Source: CAD feature listing. Evaluate the final solid. Frame: model axes, mm. Round coordinates to 2 decimals unless told otherwise and drop trailing zeros. Loops run counter-clockwise (first coordinate to the right, second up) from the corner with the lowest first, then second, coordinate; pieces in that order, holes last.
(1) Material intervals for probe 1 along Z at (x, y) = (0.2, -16.5) (3 decimals); probe 2 along Z at (x, y) = (0.85, -91.5) (3 decimals); probe 3 along Y at (x, z) = (1.05, -136), sorted ascending.
(2) Section C-C, the plane y = -9. Return the cut outline in (x, z) (3 decimals), plus the area to 3 significant figures.
(3) First-contact query: pin 1 Ø0.8 at (x, z) = (0.5, -54) entering from -Y (3 decimals); pin 2 Ø0.8 at (x, y) = (1, 13) entering from +Z (3 decimals); pin 3 Ø0.5 at (x, z) = (1, -14) entering from +Y (3 decimals). Flat tips, straight axial feed; report the tip coordinate or a pass-through.
(4) Section B-B, the plane z = -36. Return the cut outline in (x, y), plus the area to 3 significant figures.
(5) Section A-A, the plane x = 0.3. Return the cut outline in (y, z) (1 decimal).
Autodesk Inventor part; units mm, degrees
ref_plane "YZ Plane" through (0, 0, 0) normal (1, 0, 0) x (0, 1, 0)
ref_plane "XZ Plane" through (0, 0, 0) normal (0, 1, 0) x (-1, 0, 0)
ref_plane "XY Plane" through (0, 0, 0) normal (0, 0, 1) x (1, 0, 0)
sketch "Key" plane through (0, 0, 0) normal (0, 0, 1) x (1, 0, 0)
  line L0 (-9.525, 9.525) -> (9.525, 9.525) construction
  line L1 (9.525, 9.525) -> (9.525, -9.525) construction
  line L2 (9.525, -9.525) -> (-9.525, -9.525) construction
  line L3 (-9.525, -9.525) -> (-9.525, 9.525) construction
  line L4 (-9.525, 9.525) -> (9.525, -9.525) construction
  line L5 (9.525, 9.525) -> (-9.525, -9.525) construction
  point P0 (0, 0)
  point P1 (0, 0)
  dimension "d6" = 19.05
  dimension "d7" = 19.05
sketch "Col5" plane through (0, 0, 0) normal (0, 0, 1) x (1, 0, 0)
  point P0 (-10.8651, 0)
sketch "Col4" plane through (0, 0, 0) normal (0, 0, 1) x (1, 0, 0)
  point P0 (-10.8651, 0)
sketch "TC" plane through (0, 0, 0) normal (0, 0, 1) x (1, 0, 0)
  point P0 (-22.1335, 152.0917)
  dimension "d12" = 4.7625
  dimension "d13" = 4.7625
  dimension "d14" = 19.6363
sketch "Esquisse1" plane through (0, 0, 0) normal (1, 0, 0) x (0, 1, 0)
  line L0 (28.177, -71.755) -> (10.397, -71.755) construction
  line L1 (10.397, -71.755) -> (10.397, -102.235) construction
  line L2 (10.397, -102.235) -> (28.177, -102.235)
  line L3 (28.177, -102.235) -> (28.177, -71.755) construction
  line L4 (28.177, -71.755) -> (10.397, -102.235) construction
  line L5 (10.397, -71.755) -> (28.177, -102.235) construction
  line L6 (6.445, 14.065) -> (-92.805, 14.065)
  line L7 (6.445, 14.065) -> (6.445, -24.035)
  line L8 (-68.4861, -104.235) -> (30.177, -104.235)
  line L9 (30.177, -51.755) -> (30.177, -104.235)
  line L10 (-106.1694, -150.4545) -> (-142.6291, -129.4045)
  line L11 (-103.8052, -81.2096) -> (-113.3302, -97.7073)
  line L12 (-113.3302, -97.7073) -> (-117.4547, -95.3261)
  line L13 (-117.4547, -95.3261) -> (-126.9797, -111.8239)
  line L14 (-126.9797, -111.8239) -> (-131.1041, -109.4426)
  line L15 (-131.1041, -109.4426) -> (-142.6291, -129.4045)
  line L16 (-68.4861, -104.235) -> (-78.8706, -122.2214)
  line L17 (-78.8706, -122.2214) -> (-82.995, -119.8402)
  line L18 (-82.995, -119.8402) -> (-92.52, -136.338)
  line L19 (-92.52, -136.338) -> (-96.6444, -133.9567)
  line L20 (-96.6444, -133.9567) -> (-106.1694, -150.4545)
  line L21 (-92.805, 14.065) -> (-92.805, -28.035)
  line L22 (-92.805, -28.035) -> (-88.042, -28.035)
  line L23 (-88.042, -28.035) -> (-88.042, -47.085)
  line L24 (-88.042, -47.085) -> (-85.565, -47.085)
  line L25 (-85.565, -47.085) -> (-85.565, -62.135)
  line L26 (-85.565, -62.135) -> (-87.565, -62.135)
  line L27 (-89.5164, -89.4592) -> (-103.8052, -81.2096) construction
  line L28 (6.445, -24.035) -> (11.208, -24.035)
  line L29 (11.208, -24.035) -> (11.208, -43.085)
  line L30 (11.208, -43.085) -> (13.685, -43.085)
  line L31 (30.177, -51.755) -> (13.685, -43.085)
  line L32 (-78.8706, -122.2214) -> (-92.52, -136.338) construction
  line L33 (-92.52, -136.338) -> (-106.1694, -150.4545) construction
  line L34 (-103.8052, -81.2096) -> (-117.4547, -95.3261) construction
  line L35 (-131.1041, -109.4426) -> (-117.4547, -95.3261) construction
  line L36 (-103.8052, -81.2096) -> (-87.565, -81.2096)
  line L37 (-87.565, -81.2096) -> (-87.565, -62.135)
  point P0 (-5.08, 2.54)
  point P1 (19.287, -86.995)
  point P2 (-5.08, 2.54)
  point P3 (-86.042, -35.56)
  point P4 (0, 0)
extrude "Extrusion1" add sketch "Esquisse1" along normal blind 1.6
properties part number "board-profile"
Output values:
1. probe 1: z = -104.235 to 14.065
1. probe 2: z = -134.571 to -81.21, -28.035 to 14.065
1. probe 3: y = -131.21 to -97.82, -93.11 to -92.32
2. outline: (0, -104.235) - (1.6, -104.235) - (1.6, 14.065) - (0, 14.065) - close
2. area: 189 mm2
3. pin 1: stops at y = -85.565
3. pin 2: stops at z = -43.085
3. pin 3: stops at y = 6.445
4. outline: (0, -88.04) - (1.6, -88.04) - (1.6, 11.21) - (0, 11.21) - close
4. area: 159 mm2
5. outline: (-142.6, -129.4) - (-106.2, -150.5) - (-96.6, -134) - (-92.5, -136.3) - (-83, -119.8) - (-78.9, -122.2) - (-68.5, -104.2) - (30.2, -104.2) - (30.2, -51.8) - (13.7, -43.1) - (11.2, -43.1) - (11.2, -24) - (6.4, -24) - (6.4, 14.1) - (-92.8, 14.1) - (-92.8, -28) - (-88, -28) - (-88, -47.1) - (-85.6, -47.1) - (-85.6, -62.1) - (-87.6, -62.1) - (-87.6, -81.2) - (-103.8, -81.2) - (-113.3, -97.7) - (-117.5, -95.3) - (-127, -111.8) - (-131.1, -109.4) - close
